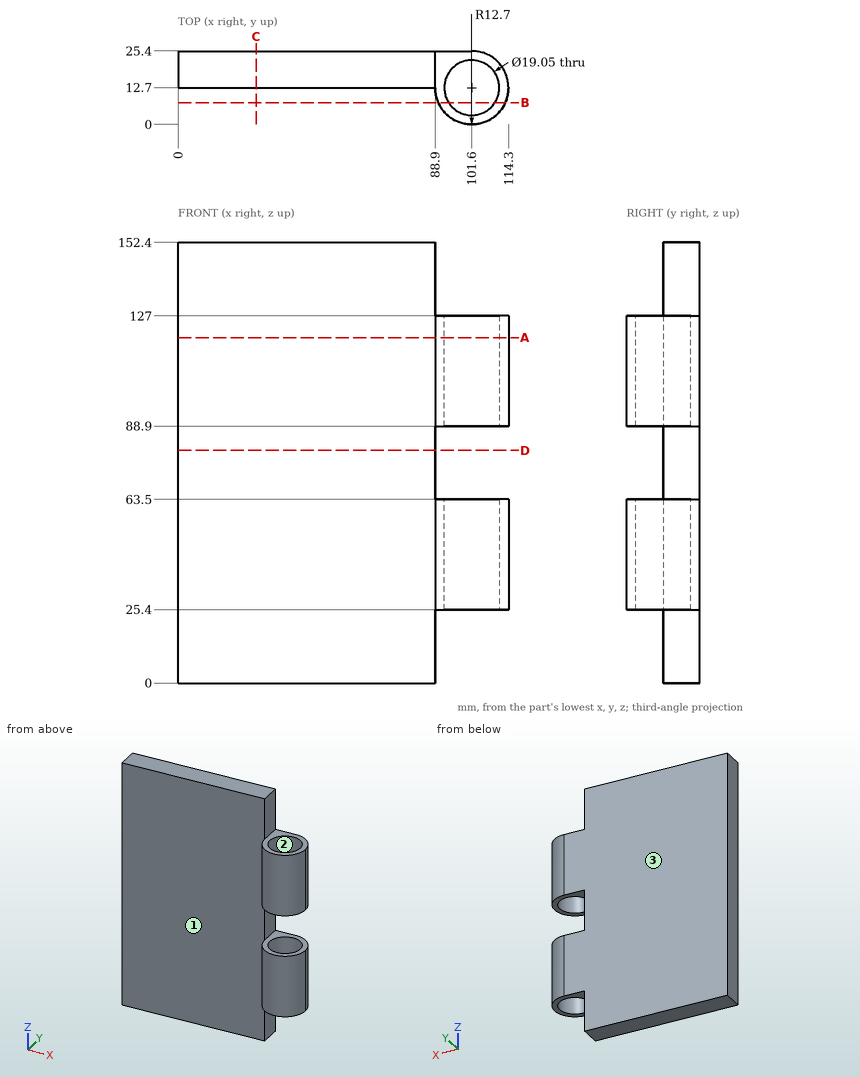
Answer from the drawing. Dimensions are ordinates in mm from the lowest x, y and z of the part. Round coordinates to 2 decimals unless told otherwise and drop trailing zeros. Write each loop counter-clockwise with the first axis right and the second up, starting at its lowest first coordinate (ties: lowest second). Pieces come first, ordered by that corner, then holes. Notation, with made-up numbers: M 62,-25.5 L 119,-25.5 A11 cw 119,-16.5 Z; hole C 10.5,2 d7. An arc over 180 degrees is marked long. Write each question's results on one line, items separated by ' | '. Start each with the question number.
Item 1: Given pin 1 Ø10 at (y, z) = (20, 140.5) entering from +X; pin 2 Ø8 at (x, z) = (41, 20) entering from -Y; pin 3 Ø6 at (y, z) = (4.5, 106) entering from +X; pin 4 Ø7.5 at (x, y) = (99, 17) entering from +Z, each flat-ended and moving along its own axis, determine where each tip first touches the part or whether it passes through.
Item 2: Find section D-D on z = 80.5. Write down the section's boundary in (x, y).
Item 3: The mould has two halves that part along Y. Classify the marked faces 1, 2 and 3: +Y half, -Y half, draft (parallel to the pull), parting line (faces both ways), or undercut.
Item 4: Find section B-B on y = 7.5. Write down the section's boundary in (x, z), and give its area (3 significant figures).
Item 5: Find section C-C on x = 27. Write down the section's boundary in (y, z).
Item 6: Straight lines are drawn through the part: probe 1 along Z at (x, y) = (97, 22); probe 2 along X at (y, z) = (13, 36.5); probe 3 along Y at (x, z) = (101, 101). For each, find the intervals that lie inside material, in ascending order.
Item 7: Find section A-A on z = 119.5. Write down the section's boundary in (x, y) (3 decimals), and give its area (3 significant figures).
Answer block:
1) pin 1: stops at x = 88.9 | pin 2: stops at y = 12.7 | pin 3: stops at x = 113.19 | pin 4: passes through
2) outline: M 0,12.7 L 88.9,12.7 L 88.9,25.4 L 0,25.4 Z
3) face 1: -Y half | face 2: undercut | face 3: +Y half
4) outline: M 90.01,25.4 L 93.62,25.4 L 93.62,63.5 L 90.01,63.5 Z; M 90.01,88.9 L 93.62,88.9 L 93.62,127 L 90.01,127 Z; M 109.58,25.4 L 113.19,25.4 L 113.19,63.5 L 109.58,63.5 Z; M 109.58,88.9 L 113.19,88.9 L 113.19,127 L 109.58,127 Z | area: 550 mm²
5) outline: M 12.7,0 L 25.4,0 L 25.4,152.4 L 12.7,152.4 Z
6) probe 1: z = 25.4 to 63.5, 88.9 to 127 | probe 2: x = 0 to 92.08, 111.12 to 114.3 | probe 3: y = 0.01 to 3.19, 22.21 to 25.4
7) outline: M 0,12.7 L 88.9,12.7 A12.7 ccw long 101.6,25.4 L 0,25.4 Z; hole C 101.6,12.7 d19.05 | area: 1,390 mm²
